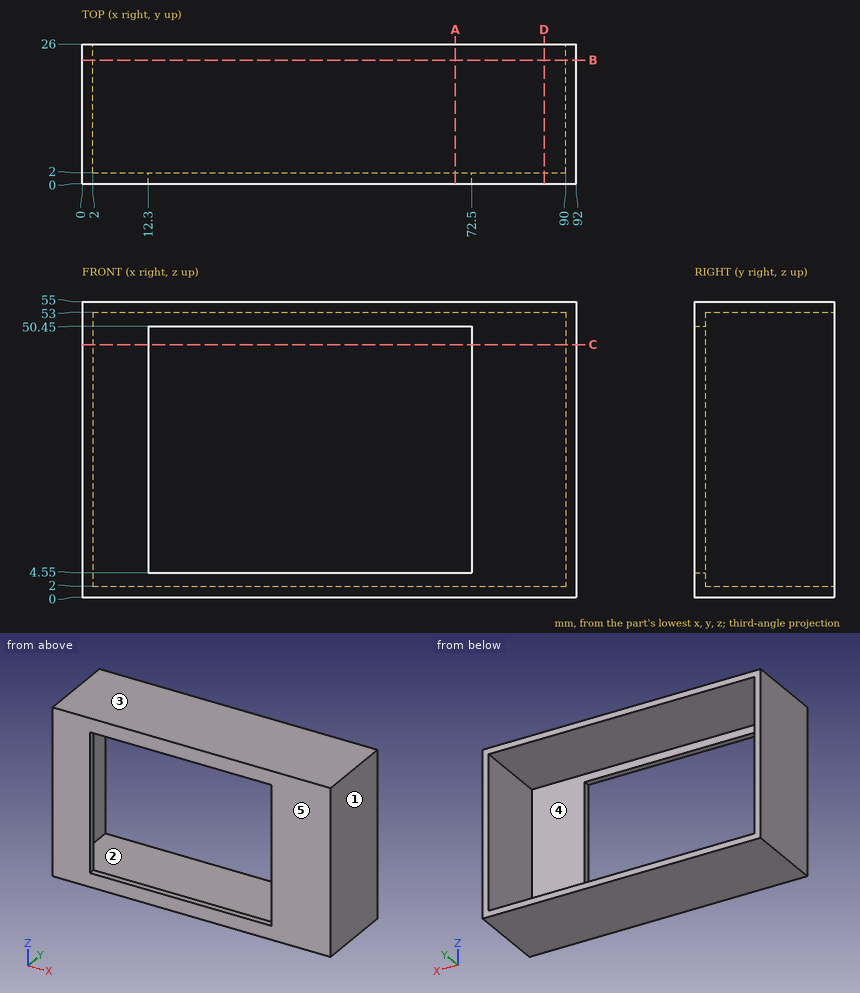
Source: three-view drawing plus pictorial views. Frame: mm from the lowest corner of the part. A direction names the side the tool comes from. Round coordinates to 2 decimals unless told otherwise and drop trailing zeros. Loops run counter-clockwise (first coordinate to the right, second up) from the corner with the lowest first, then second, coordinate; pieces in that order, holes last. Notation, with made-up numbers: (51.25, 3.25) - (110.25, 3.25) arc R34 cw to (110.25, 36.25) - close; hole circle Ø9 at (-28, 87.5). An arc over 180 degrees is marked (long way). Write each question's results on one line, items separated by ' | '. Start each with the question number.
1) Line query: probe 1 along Z at (x, y) = (64, 5.25); probe 2 along X at (y, z) = (6, 30.5); probe 3 along X at (y, z) = (1.5, 11). Output: solid intervals per line, ascending. Write a range as [from, to].
2) Cut plane C-C on z = 47. Return loops of the section in (x, y).
3) Cut plane B-B on y = 23. Return loops of the section in (x, z).
4) Mould query, pull axis Z, two halves, no side actions, for the marked faces 3, 4 and 5. Classes: released by +Z, released by -Z, zero draft, split by the parting line, or undercut.
5) Cut plane D-D on x = 86. Return loops of the section in (y, z), then the cut area to 3 significant figures.
6) Cut plane A-A on x = 69.5. Return loops of the section in (y, z).
7) Access query for the marked faces 1 and 2. Directions: +Z, -Z, +X, -X, +Y, -Y. A direction counts if a zero-diameter tool reaches every point of the face in a straight line with its end or side. Return the directions, or none.
8) First-contact query: P1, Ø10, axis at x = 53, z = 14, coming from the +Y side. Flat tip, straight axial feed; report the tip coordinate or a pass-through.
Verdict:
1) probe 1: z = [0, 2], [53, 55] | probe 2: x = [0, 2], [90, 92] | probe 3: x = [0, 12.3], [72.5, 92]
2) outline: (0, 0) - (12.3, 0) - (12.3, 2) - (2, 2) - (2, 26) - (0, 26) - close; (72.5, 0) - (92, 0) - (92, 26) - (90, 26) - (90, 2) - (72.5, 2) - close
3) outline: (0, 0) - (92, 0) - (92, 55) - (0, 55) - close; hole (2, 2) - (90, 2) - (90, 53) - (2, 53) - close
4) face 3: released by +Z | face 4: undercut | face 5: zero draft
5) outline: (0, 0) - (26, 0) - (26, 2) - (2, 2) - (2, 53) - (26, 53) - (26, 55) - (0, 55) - close | area: 206 mm2
6) outline: (0, 0) - (26, 0) - (26, 2) - (2, 2) - (2, 4.55) - (0, 4.55) - close; (0, 50.45) - (2, 50.45) - (2, 53) - (26, 53) - (26, 55) - (0, 55) - close
7) face 1: +Z, -Z, +X, +Y, -Y | face 2: +Y
8) P1: passes through
